Build history of the part. All positions in model axes, mm. A direction names the side the tool comes from. Coordinates: 2 decimals unless noted, no trailing zeros. Order: outer loops, then holes, each group sorted by start corner. A loop starts at its lowest first (then second) coordinate and runs counter-clockwise, first axis right, second up. Notation, with made-up numbers: (37, -34) - (57, -34) arc R32 cw to (57, -2) - close; hole circle Ø9 at (78, 49.5). An arc over 180 degrees is marked (long way). Return JSON: item names as keys, results as strings.
from build123d import *

# Parameters (mm, degrees)
BOSS_EXTRUDE1_DEPTH = 0.2
BOSS_EXTRUDE2_DEPTH = 12.58
SKETCH1_8_W         = 162.49
SKETCH1_8_H         = 1
BOSS_EXTRUDE3_DEPTH = 15.58
BOSS_EXTRUDE4_DEPTH = 12.38
BOSS_EXTRUDE5_DEPTH = 2.58


with BuildPart() as part:
    # Sketch1 → Boss-Extrude1 (new body)
    with BuildSketch(Plane(origin=(0, 0, 0), x_dir=(1, 0, 0), z_dir=(0, 1, 0))):
        Polygon((-113.845299462, 0), (-110.422649731, -5.92820323), (110.422649731, -5.92820323), (113.845299462, 0), (3.422649731, 191.25763964), (-3.422649731, 191.25763964), align=None)
        Polygon((108.979274058, -3.42820323), (-108.979274058, -3.42820323), (-110.958548116, 0), (-1.979274058, 188.75763964), (1.979274058, 188.75763964), (110.958548116, 0), align=None, mode=Mode.SUBTRACT)
    extrude(amount=BOSS_EXTRUDE1_DEPTH)

    # Sketch1<7> → Boss-Extrude2 (add)
    with BuildSketch(Plane(origin=(0, 0, 0), x_dir=(1, 0, 0), z_dir=(0, 1, 0))):
        Polygon((-95.137949192, 30.402081141), (-96.003974596, 30.902081141), (-113.845299462, 0), (-110.422649731, -5.92820323), (-74.74, -5.92820323), (-74.74, -4.92820323), (-109.845299462, -4.92820323), (-112.690598923, 0), align=None)
        Polygon((-3.422649731, 191.25763964), (-14.758974596, 171.622549002), (-13.892949192, 171.122549002), (-2.845299462, 190.25763964), (2.845299462, 190.25763964), (13.892949192, 171.122549002), (14.758974596, 171.622549002), (3.422649731, 191.25763964), align=None)
        Polygon((109.845299462, -4.92820323), (87.75, -4.92820323), (87.75, -5.92820323), (110.422649731, -5.92820323), (113.845299462, 0), (102.508974596, 19.635090638), (101.642949192, 19.135090638), (112.690598923, 0), align=None)
        Polygon((61.133974596, 91.298692801), (56.133974596, 99.958946839), (55.267949192, 99.458946839), (60.267949192, 90.798692801), align=None)
    extrude(amount=BOSS_EXTRUDE2_DEPTH)

    # Sketch1<8> → Boss-Extrude3 (add)
    with BuildSketch(Plane(origin=(0, 0, 0), x_dir=(1, 0, 0), z_dir=(0, 1, 0))):
        Polygon((-14.758974596, 171.622549002), (-96.003974596, 30.902081141), (-95.137949192, 30.402081141), (-13.892949192, 171.122549002), align=None)
        with Locations((6.505, -5.42820323)):
            Rectangle(SKETCH1_8_W, SKETCH1_8_H)
        Polygon((56.133974596, 99.958946839), (14.758974596, 171.622549002), (13.892949192, 171.122549002), (55.267949192, 99.458946839), align=None)
        Polygon((102.508974596, 19.635090638), (61.133974596, 91.298692801), (60.267949192, 90.798692801), (101.642949192, 19.135090638), align=None)
    extrude(amount=BOSS_EXTRUDE3_DEPTH)

    # Sketch1<9> → Boss-Extrude4 (add)
    with BuildSketch(Plane(origin=(0, 0, 0), x_dir=(1, 0, 0), z_dir=(0, 1, 0))):
        Polygon((-112.113248654, 0), (-110.834936491, -2.214101615), (-109.556624327, -4.42820323), (109.556624327, -4.42820323), (112.113248654, 0), (2.556624327, 189.75763964), (-2.556624327, 189.75763964), align=None)
        Polygon((-110.958548116, 0), (-56.468911087, 94.37881982), (-1.979274058, 188.75763964), (1.979274058, 188.75763964), (110.958548116, 0), (108.979274058, -3.42820323), (-108.979274058, -3.42820323), align=None, mode=Mode.SUBTRACT)
    extrude(amount=-BOSS_EXTRUDE4_DEPTH)

    # Sketch1<10> → Boss-Extrude5 (add)
    with BuildSketch(Plane(origin=(0, 0, 0), x_dir=(1, 0, 0), z_dir=(0, 1, 0))):
        Polygon((61.133974596, 91.298692801), (56.133974596, 99.958946839), (55.267949192, 99.458946839), (60.267949192, 90.798692801), align=None)
    extrude(amount=-BOSS_EXTRUDE5_DEPTH)


solid = part.part
1. Tool access for faces 4 (the flat face through (-56.568, -6.103, -96.207)), 5 (the flat face through (58, 0.2, -93)), 6 (the flat face through (57.733, -1.272, -95.189)), 7 (the flat face through (58, -2.58, -95.4)), 8 (the flat face through (-57.23, -6, -93.06)): list every direction of +Z, -Z, +X, -X, +Y, -Y with a clear straight run to the whole face (end or side of a thin tool).
Check values:
{"face 4": "-Z, -X, -Y", "face 5": "+Y", "face 6": "-Y", "face 7": "-Z, +X, -Y", "face 8": "+Y, -Y"}
2. Cut at D-D on y = 4. Give the cut face in (x, z).
Check values:
{"outline": "(-113.85, 0) - (-3.42, -191.26) - (3.42, -191.26) - (113.85, 0) - (110.42, 5.93) - (-110.42, 5.93) - close; hole (-112.69, 0) - (-2.85, -190.26) - (2.85, -190.26) - (112.69, 0) - (109.85, 4.93) - (-109.85, 4.93) - close"}
3. Cut at B-B on z = -61. Give the cut face in (x, y), plus the area to 3 significant figures.
Check values:
{"outline": "(-78.63, 0) - (-76.89, 0) - (-76.89, -12.38) - (-75.74, -12.38) - (-75.74, 0.2) - (-77.47, 0.2) - (-77.47, 15.58) - (-78.63, 15.58) - close; (75.74, -12.38) - (76.89, -12.38) - (76.89, 0) - (78.63, 0) - (78.63, 15.58) - (77.47, 15.58) - (77.47, 0.2) - (75.74, 0.2) - close", "area": "65.3 mm²"}
4. Mould opens along Z. For faces 1 (the flat face through (-6, 12.58, -186)), 2 (the flat face through (-111.248, 6.303, 2.499)), 3 (the flat face through (-2, -6, 4.428)) say: pulls with the +Z half, pulls with the -Z half, needs draft (parallel to the pull), parting line crosses it, or undercut.
Check values:
{"face 1": "needs draft", "face 2": "undercut", "face 3": "pulls with the +Z half"}
5. Cut at A-A on y = -9.75. Give the cut face in (x, z), plus the area to 3 significant figures.
Check values:
{"outline": "(-112.11, 0) - (-2.56, -189.76) - (2.56, -189.76) - (112.11, 0) - (109.56, 4.43) - (-109.56, 4.43) - close; hole (-110.96, 0) - (-1.98, -188.76) - (1.98, -188.76) - (110.96, 0) - (108.98, 3.43) - (-108.98, 3.43) - close", "area": "669 mm²"}
6. Drop flat-ended pins along their axis: pin 1 (1 mm diameter, centred on y = 5, z = -66, fed in from -X); pin 2 (3 mm diameter, centred on x = -1, y = -3, fed in from +Z); pin 3 (8 mm diameter, centred on y = 2, z = -24.5, fed in from +X). Give the stop position or say it passes through.
Check values:
{"pin 1": "x = -76.03", "pin 2": "z = 4.43", "pin 3": "x = 102.01"}
7. Cut at C-C on x = -60. Give the cut face in (y, z).
Check values:
{"outline": "(-12.38, -90.26) - (0, -90.26) - (0, -93.26) - (15.58, -93.26) - (15.58, -91.26) - (0.2, -91.26) - (0.2, -88.26) - (-12.38, -88.26) - close; (-12.38, 3.43) - (0.2, 3.43) - (0.2, 4.93) - (15.58, 4.93) - (15.58, 5.93) - (0, 5.93) - (0, 4.43) - (-12.38, 4.43) - close"}
8. Probe L1, parallel to Z at x = -70.5, y = 9.75; L2, parallel to X at y = 7, z = -45; L3, parallel to Z at x = 56, y = -3.75. List the from-to ranges inside material, lowest first.
Check values:
{"L1": "-75.08 to -73.08, 4.93 to 5.93", "L2": "-87.86 to -86.71, 86.71 to 87.86", "L3": "-97.19 to -95.19, 3.43 to 4.43"}
